Here's the drawing with two shaded views (mm, measured from the low corner). I have some questions. Round coordinates to 2 decimals unless told otherwise and drop trailing zeros. Loops run counter-clockwise (first coordinate to the right, second up) from the corner with the lowest first, then second, coordinate; pieces in that order, holes last. Notation, with made-up numbers: M 87.25,-35 L 133.25,-35 A11 cw 133.25,-20 Z; hole C 87.25,8.25 d2. An arc over 180 degrees is marked long. Answer as CSV lines item,"result".
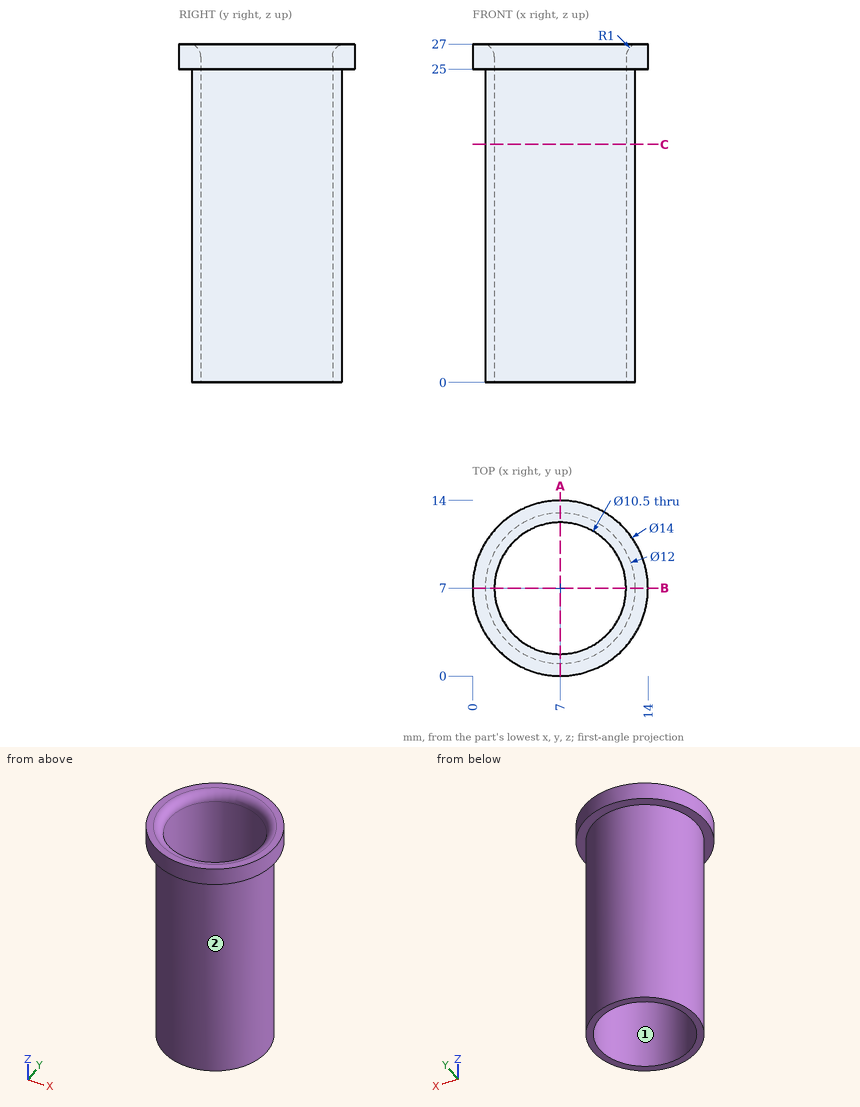
1. We'd pull the mould along X, two halves only. Please class the marked faces 1 and 2: pulls with the +X half, pulls with the -X half, needs draft (parallel to the pull), parting line crosses it, or undercut.
Evaluation:
face 1,"undercut"
face 2,"parting line crosses it"
2. I want a section at A-A, the plane x = 7. Please give me the cut outline in (y, z), and give its area (3 significant figures).
Evaluation:
outline,"M 0,25 L 1,25 L 1,0 L 1.75,0 L 1.75,26 A1 ccw 0.75,27 L 0,27 Z; M 12.25,0 L 13,0 L 13,25 L 14,25 L 14,27 L 13.25,27 A1 ccw 12.25,26 Z"
area,"44.1 mm²"
3. If I drill on line 1 (Y direction, x = 7, z = 16.25); line 2 (Z direction, x = 7.25, y = 13.25); line 3 (Y direction, x = 10.25, z = 17.5), over which ranges is the centre line in solid material (lowest first)? Write a range as [from, to].
Evaluation:
line 1,"y = [1, 1.75], [12.25, 13]"
line 2,"z = [25, 27]"
line 3,"y = [1.96, 2.88], [11.12, 12.04]"
4. For P1, Ø4, axis at y = 12.5, z = 23.5, coming from the -X side; P2, Ø4, axis at y = 6, z = 22.5, coming from the +X side; P3, Ø7, axis at x = 4.5, y = 9.5, coming from the -Z side; P4, Ø3, axis at x = 6, z = 21, coming from the -Y side, each with a flat end and sliding along its axis, tell me the tip position at first contact or that it passes through.
Evaluation:
P1,"stops at x = 1.38"
P2,"stops at x = 13"
P3,"stops at z = 0"
P4,"stops at y = 1"
5. I want a section at C-C, the plane z = 19. Please give me the cut outline in (x, y).
Evaluation:
outline,"C 7,7 d12; hole C 7,7 d10.5"
